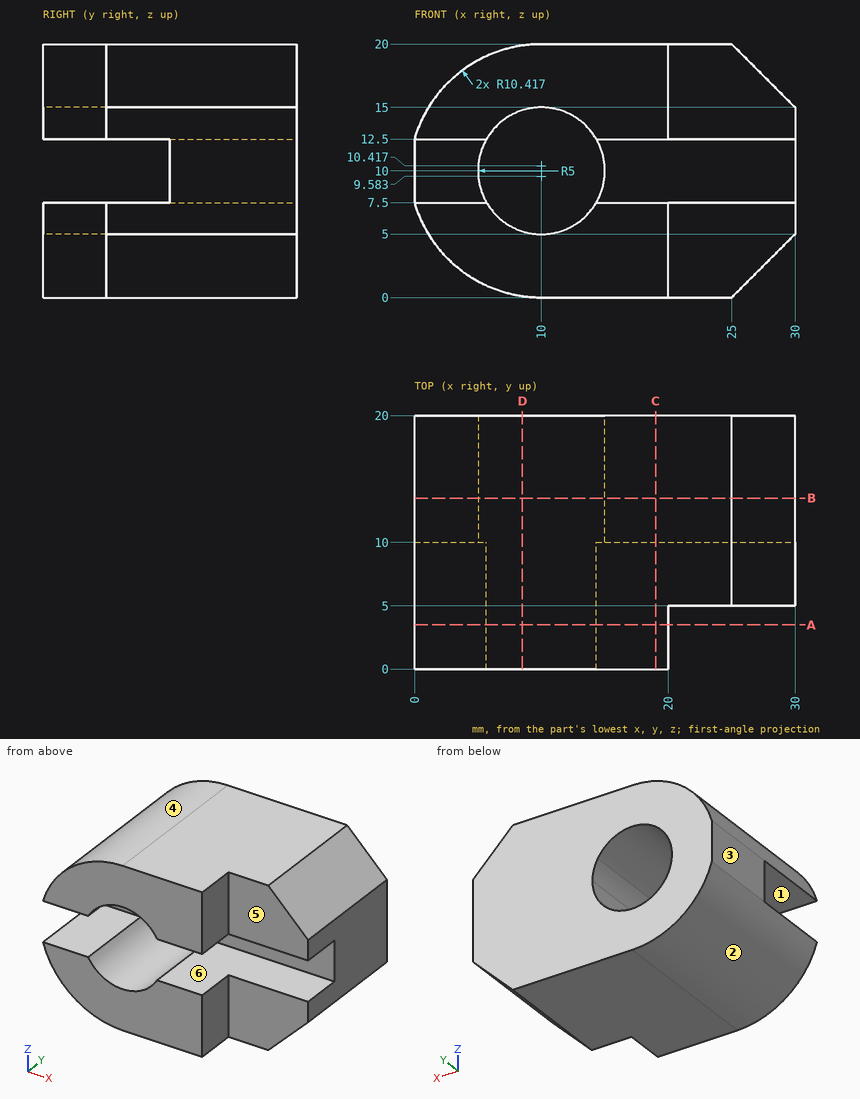
Geometry check sheet. Reference: drawing and pictorial views, mm from the part's lowest x, y, z. A direction names the side the tool comes from. Round coordinates to 2 decimals unless told otherwise and drop trailing zeros. Order: outer loops, then holes, each group sorted by start corner. A loop starts at its lowest first (then second) coordinate and runs counter-clockwise, first axis right, second up. Notation, with made-up numbers: M 30,84.25 L 73,84.25 A18 ccw 73,106.25 Z; hole C 86,45.5 d9. An arc over 180 degrees is marked long. One line per item, written item: value. Start each with the question number.
1. Section check A-A on y = 3.5. Enter the section's corners in (x, z).
2. Section check B-B on y = 13.5. Enter the section's corners in (x, z), and give its area (3 significant figures).
3. Section check D-D on x = 8.5. Enter the section's corners in (y, z), and give its area (3 significant figures).
4. Section check C-C on x = 19. Enter the section's corners in (y, z).
5. Release check for a two-part mould opening along Z. For the marked faces 1, 2 and 3 record: released by +Z, released by -Z, zero draft, split by the parting line, or undercut.
6. Access from +Z, -Z, +X, -X, +Y, -Y to the whole of each face (thin tool, end or side, straight path). Record for the marked faces 4, 5 and 6.
7. Gauge pin test, flat ends, axial feed: P1, Ø1.7, axis at x = 3.5, y = 3.5, coming from the +Z side (1 decimal); P2, Ø4.5, axis at x = 2.5, y = 3.5, coming from the -Z side; P3, Ø5, axis at y = 5, z = 16.5, coming from the -X side. Record the tip position at first contact, or that the pin passes through.
8. Scan lines: line 1 along Z through (x, y) = (22, 9.5); line 2 along Y through (x, z) = (24, 6.5); line 3 along Z through (x, y) = (8.5, 13). Record each from-to range of solid material in increasing order.
Results found:
1. outline: M 0,7.5 A10.42 ccw 10,0 L 20,0 L 20,7.5 L 14.33,7.5 A5 cw 5.67,7.5 Z; M 0,12.5 L 5.67,12.5 A5 cw 14.33,12.5 L 20,12.5 L 20,20 L 10,20 A10.42 ccw Z
2. outline: M 0,7.5 A10.42 ccw 10,0 L 25,0 L 30,5 L 30,15 L 25,20 L 10,20 A10.42 ccw 0,12.5 Z; hole M 14.33,7.5 A5 ccw 15,10 A5 ccw 14.33,12.5 A5 ccw long Z
2. area: 457 mm^2
3. outline: M 0,0.11 L 20,0.11 L 20,5.23 L 0,5.23 Z; M 0,14.77 L 20,14.77 L 20,19.89 L 0,19.89 Z
3. area: 205 mm^2
4. outline: M 0,0 L 20,0 L 20,20 L 0,20 L 0,12.5 L 10,12.5 L 10,7.5 L 0,7.5 Z
5. face 1: undercut
5. face 2: released by -Z
5. face 3: zero draft
6. face 4: +Z, -X, +Y, -Y
6. face 5: +Z, -Z, +X, -Y
6. face 6: +X, -X, -Y
7. P1: z = 18.3
7. P2: z = 1.42
7. P3: x = 0.57
8. line 1: 0 to 7.5, 12.5 to 20
8. line 2: 5 to 20
8. line 3: 0.11 to 5.23, 14.77 to 19.89
